The listing builds one solid part. Answer for the finished solid, in the listing's coordinates (mm). Face numbers are marked on the shaded views. Round coordinates to 2 decimals unless told otherwise and drop trailing zeros. Write each loop counter-clockwise with the first axis right and the second up, starting at its lowest first coordinate (ties: lowest second). Pieces come first, ordered by that corner, then holes.
(1) This flat-tipped pin is pushed along its axis until it touches: pin 1 Ø4 at (x, z) = (19, 101) entering from -Y. Where does it stop, or does it pass through?
(2) A cutting plane is placed at A-A, the plane x = 15.5. Give the vertices of the cut face in (y, z).
(3) Find the intervals of material crossed by probe 1 along Y at (x, z) = (13, 87); probe 2 along Z at (x, y) = (5, -369.5); probe 3 along Y at (x, z) = (3.5, 102.75), in increasing order.
(4) A cutting plane is placed at B-B, the plane z = 99.25. Give the vertices of the cut face in (x, y).
(5) The mould has two halves that part along Z. Classify the marked faces 1, 2 and 3: +Z half, -Z half, draft (parallel to the pull), parting line (faces both ways), or undercut.
from build123d import *

# Parameters (mm, degrees)
BOSS_EXTRUDE1_DEPTH = 26
SKETCH4_R           = 8.5
CUT_EXTRUDE1_DEPTH  = 33
FILLET1_R           = 13
SKETCH5_R           = 11
SKETCH5_R_2         = 8.5
BOSS_EXTRUDE2_DEPTH = 8


with BuildPart() as part:
    # Sketch3 → Boss-Extrude1 (new body)
    with BuildSketch(Plane(origin=(0, 0, 0), x_dir=(0, 0, -1), z_dir=(1, 0, 0))):
        Polygon((-91.872113318, -345.981347093), (-105.872113318, -345.981347093), (-105.872113318, -400.567582276), (-112.872113318, -400.567582276), (-112.872113318, -369.669881287), (-112.872113318, -119.459461353), (-84.872113318, -119.459461353), (-84.872113318, -369.669881287), (-84.872113318, -400.882361345), (-91.872113318, -400.882361345), align=None)
    extrude(amount=BOSS_EXTRUDE1_DEPTH)

    # Sketch4 → Cut-Extrude1 (cut)
    with BuildSketch(Plane.XY.offset(112.872113318)):
        with Locations((13, -387.882361345)):
            Circle(SKETCH4_R)
    extrude(amount=-CUT_EXTRUDE1_DEPTH, mode=Mode.SUBTRACT)

    # Fillet1
    fillet1_edges = [part.edges().sort_by_distance(p)[0] for p in [
        (26, -400.567582276, 109.372113318),
        (26, -400.882361345, 88.372113318),
        (0, -400.567582276, 109.372113318),
        (0, -400.882361345, 88.372113318),
    ]]
    fillet(fillet1_edges, radius=FILLET1_R - 0.0001)  # a hair under: the kernel refuses the full size

    # Sketch5 → Boss-Extrude2 (add)
    with BuildSketch(Plane.XY.offset(112.872113318)):
        with Locations((13, -387.882361345)):
            Circle(SKETCH5_R)
        with Locations((13, -387.882361345)):
            Circle(SKETCH5_R_2, mode=Mode.SUBTRACT)
    boss_extrude2 = extrude(amount=-BOSS_EXTRUDE2_DEPTH)

    # Mirror1: Boss-Extrude2 across plane
    add(boss_extrude2.mirror(Plane.XY.offset(98.872113318)))


solid = part.part
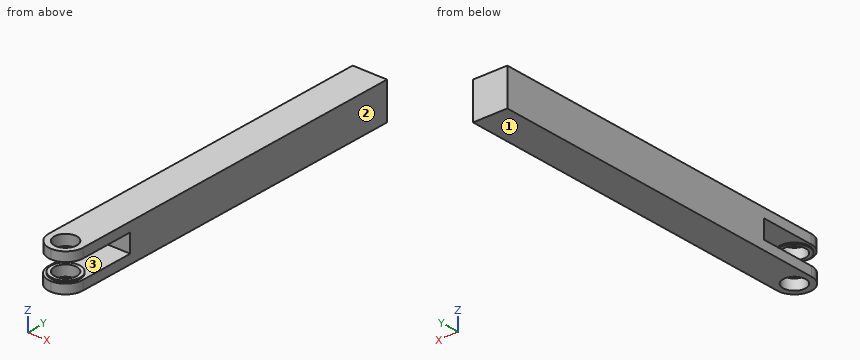
Solutions:
1. pin 1: stops at y = -345.98
2. outline: (-400.64, 84.87) - (-396.01, 84.87) - (-396.01, 92.87) - (-398.59, 92.87) - (-398.59, 91.87) - (-400.64, 91.87) - close; (-400.32, 105.87) - (-398.59, 105.87) - (-398.59, 104.87) - (-396.01, 104.87) - (-396.01, 112.87) - (-400.32, 112.87) - close; (-379.76, 84.87) - (-119.46, 84.87) - (-119.46, 112.87) - (-379.76, 112.87) - (-379.76, 104.87) - (-377.17, 104.87) - (-377.17, 105.87) - (-345.98, 105.87) - (-345.98, 91.87) - (-377.17, 91.87) - (-377.17, 92.87) - (-379.76, 92.87) - close
3. probe 1: y = -400.88 to -396.38, -379.38 to -119.46
3. probe 2: z = 84.87 to 91.87, 105.87 to 112.87
3. probe 3: y = -345.98 to -119.46
4. outline: (0, -345.98) - (26, -345.98) - (26, -119.46) - (0, -119.46) - close
5. face 1: -Z half
5. face 2: draft
5. face 3: undercut
